Input: part model. Units: mm. Frame: model coordinates. A direction names the side the tool comes from. Round coordinates to 2 decimals unless told otherwise and drop trailing zeros. Loops run counter-clockwise (first coordinate to the right, second up) from the corner with the lowest first, then second, coordinate; pieces in that order, holes last. Notation, with made-up numbers: M 63.5,29.5 L 120.5,29.5 A18 cw 120.5,57.5 Z; hole C 38.25,26.5 d7. An arc over 180 degrees is marked long. Return JSON: item names as keys, results as strings. Group by question number.
1) Section A-A (y = 21.75). Output: boundary loops of the cut face in (x, z), plus the area to 3 significant figures.
2) Section C-C (x = -21). Output: boundary loops of the cut face in (y, z), plus the area to 3 significant figures.
3) Material intervals for line 1 (Y direction, x = -4.25, z = 12); line 2 (Z direction, x = -4.25, y = 11.25); line 3 (Z direction, x = -14.75, y = 13), sorted ascending. Write a range as from..to.
4) Mould query, pull axis Z, two halves, no side actions, for faces 1 (the face through (-8, 14, 0)), 2 (the face through (-15, 0, -7)), 3 (the face through (-12, 13, -15)). Classes: +Z half, -Z half, draft (parallel to the pull), parting line (faces both ways), or undercut.
5) Section B-B (y = 13.5). Output: boundary loops of the cut face in (x, z).
6) Section D-D (x = -14.75). Output: boundary loops of the cut face in (y, z).
7) Access query for faces 4 (the face through (-22.25, 3.45, -0.15)), 5 (the face through (-25, 13, 0)), 6 (the face through (-6.1, 24, -1.2)). Directions: +Z, -Z, +X, -X, +Y, -Y. A direction counts if a zero-diameter tool reaches every point of the face in a straight line with its end or side. Return the directions, or none.
from build123d import *

# Parameters (mm, degrees)
SKETCH1_R            = 7
SKETCH1_R_2          = 2.75
SKETCH1_R_3          = 3.659852489
BOSS_EXTRUDE1_DEPTH  = 7
SKETCH2_R            = 8
SKETCH2_R_2          = 6
BOSS_EXTRUDE2_DEPTH  = 17
FILLET1_R            = 3
FILLET2_R            = 3
SKETCH3_R            = 1
SKETCH5_W            = 50
SKETCH5_H            = 30
BOSS_EXTRUDE3_DEPTH  = 27
SKETCH6_R            = 2
CUT_EXTRUDE1_DEPTH   = 57
INTERSECT3_OUTLINE_W = 27
INTERSECT3_OUTLINE_H = 30
INTERSECT3_OUTLINE_R = 2
INTERSECT3_DEPTH     = 25


with BuildPart() as part:
    # Sketch1 → Boss-Extrude1 (new body)
    with BuildSketch(Plane(origin=(0, 0, 0), x_dir=(1, 0, 0), z_dir=(0, 1, 0))):
        with BuildLine():
            ThreePointArc((-15.634333704, 6.748663161), (-22.25, 0), (-15.634333704, -6.748663161))
            ThreePointArc((-15.634333704, -6.748663161), (-12.054001616, -7.488359295), (-8.978814065, -9.465516285))
            ThreePointArc((-8.978814065, -9.465516285), (-0.448762307, -12.99442036), (8.273320847, -9.971141939))
            ThreePointArc((8.273320847, -9.971141939), (11.493139678, -8.165901558), (15.148520579, -7.651784261))
            ThreePointArc((15.148520579, -7.651784261), (23.159852489, 0), (15.148520579, 7.651784261))
            ThreePointArc((15.148520579, 7.651784261), (11.493139678, 8.165901558), (8.273320847, 9.971141939))
            ThreePointArc((8.273320847, 9.971141939), (-0.448762307, 12.99442036), (-8.978814065, 9.465516285))
            ThreePointArc((-8.978814065, 9.465516285), (-12.054001616, 7.488359295), (-15.634333704, 6.748663161))
        make_face()
        with Locations(Location((0, 0, 0), (0, 0, 270))):
            Circle(SKETCH1_R, mode=Mode.SUBTRACT)
        with Locations(Location((-15.5, 0, 0), (0, 0, 270))):
            Circle(SKETCH1_R_2, mode=Mode.SUBTRACT)
        with Locations(Location((15.5, 0, 0), (0, 0, 270))):
            Circle(SKETCH1_R_3, mode=Mode.SUBTRACT)
    extrude(amount=BOSS_EXTRUDE1_DEPTH)

    # Sketch2 → Boss-Extrude2 (add)
    with BuildSketch(Plane(origin=(0, 7, 0), x_dir=(1, 0, 0), z_dir=(0, 1, 0))):
        with Locations(Location((0, 0, 0), (0, 0, 270))):
            Circle(SKETCH2_R)
        with Locations(Location((0, 0, 0), (0, 0, 270))):
            Circle(SKETCH2_R_2, mode=Mode.SUBTRACT)
    extrude(amount=BOSS_EXTRUDE2_DEPTH)

    # Fillet1
    # the kernel refuses this fillet: 3 mm, written as the material it adds along each edge
    with BuildSketch(Plane(origin=(0, 7, 0), x_dir=(0, 0, 1), z_dir=(-1, 0, 0))) as fillet1_piece_1:
        with BuildLine():
            CenterArc((4, -2.236067977), FILLET1_R, 0, 48.189685104)
            Line((6, 0), (6.04, 0.04472136))
            ThreePointArc((6.04, 0.04472136), (6.5, 0.06), (7, 0.06))
            Line((7, 0.06), (7.06, 0))
            Line((7.06, 0), (7.06, -2.236067977))
            Line((7.06, -2.236067977), (7, -2.236067977))
        make_face()
    revolve(axis=Axis((0, 7, 0), (0, 1, 0)))
    with BuildSketch(Plane(origin=(0, 7, 0), x_dir=(0, 0, 1), z_dir=(-1, 0, 0))) as fillet1_piece_2:
        with BuildLine():
            CenterArc((8 + FILLET1_R, FILLET1_R), FILLET1_R, 180, 90)
            Line((8, FILLET1_R), (8 - FILLET1_R * 0.02, FILLET1_R))
            Line((8 - FILLET1_R * 0.02, FILLET1_R), (8 - FILLET1_R * 0.02, -FILLET1_R * 0.02))
            Line((8 - FILLET1_R * 0.02, -FILLET1_R * 0.02), (8 + FILLET1_R, -FILLET1_R * 0.02))
            Line((8 + FILLET1_R, -FILLET1_R * 0.02), (8 + FILLET1_R, 0))
        make_face()
    revolve(axis=Axis((0, 7, 0), (0, 1, 0)))

    # Fillet2
    fillet2_edges = [part.edges().sort_by_distance(p)[0] for p in [
        (0, 7, -6),
    ]]
    fillet(fillet2_edges, radius=FILLET2_R)


with BuildPart() as body_2:
    # Sketch3 → Revolve1 (revolve)
    with BuildSketch(Plane(origin=(0, 0, 0), x_dir=(0, 0, -1), z_dir=(1, 0, 0))):
        with Locations((8.5, 19.608844607)):
            Circle(SKETCH3_R)
    revolve(axis=Axis((0, 0, 0), (0, 1, 0)))


with BuildPart() as part_1:
    add(part.part)

    # Intersect1: read off the stored shape, not the designer's step
    # Intersect1: cut body 2
    add(body_2.part, mode=Mode.SUBTRACT)


with BuildPart() as body_2_2:
    # Sketch5 → Boss-Extrude3 (new body)
    with BuildSketch(Plane(origin=(0, 0, 0), x_dir=(-1, 0, 0), z_dir=(0, -1, 0))):
        Rectangle(SKETCH5_W, SKETCH5_H)
    extrude(amount=-BOSS_EXTRUDE3_DEPTH)

    # Sketch6 → Cut-Extrude1 (cut)
    with BuildSketch(Plane.ZY.offset(25)):
        with Locations((-11.920412871, 13.5)):
            Circle(SKETCH6_R)
        with Locations(Location((11.920412871, 13.5, 0), (0, 0, 180))):
            Circle(SKETCH6_R)
    extrude(amount=-CUT_EXTRUDE1_DEPTH, mode=Mode.SUBTRACT)

    # Intersect2: read off the stored shape, not the designer's step
    # Intersect2: cut part
    add(part_1.part, mode=Mode.SUBTRACT)

    # Intersect3: read off the stored shape, not the designer's step
    # Intersect3 outline → Intersect3 (cut)
    with BuildSketch(Plane.YZ):
        with Locations((13.5, 0)):
            Rectangle(INTERSECT3_OUTLINE_W, INTERSECT3_OUTLINE_H)
        with Locations((13.5, -11.920412871)):
            Circle(INTERSECT3_OUTLINE_R, mode=Mode.SUBTRACT)
        with Locations((13.5, 11.920412871)):
            Circle(INTERSECT3_OUTLINE_R, mode=Mode.SUBTRACT)
    extrude(amount=INTERSECT3_DEPTH, mode=Mode.SUBTRACT)


solid = body_2_2.part
Returned:
{
 "1": {"outline": "M -25,-15 L 0,-15 L 0,-8 A8 cw 0,8 L 0,15 L -25,15 Z; M 0,-6 L 0,6 A6 ccw Z", "area": "706 mm^2"},
 "2": {"outline": "M 0,-15 L 27,-15 L 27,15 L 0,15 L 0,3.91 L 7,3.91 L 7,-3.91 L 0,-3.91 Z; hole C 13.5,-11.92 d4; hole C 13.5,11.92 d4", "area": "730 mm^2"},
 "3": {"line 1": "y = 7..11.5, 15.5..27", "line 2": "z = -15..-6.78, -4.24..4.24, 6.78..15", "line 3": "z = -15..-13.86, -9.98..9.98, 13.86..15"},
 "4": {"face 1": "undercut", "face 2": "draft", "face 3": "-Z half"},
 "5": {"outline": "M -25,-15 L 0,-15 L 0,-13.92 L -25,-13.92 Z; M -25,-9.92 L 0,-9.92 L 0,-8 A8 cw 0,8 L 0,9.92 L -25,9.92 Z; M -25,13.92 L 0,13.92 L 0,15 L -25,15 Z; M 0,-6 L 0,6 A6 ccw Z"},
 "6": {"outline": "M 0,-15 L 27,-15 L 27,15 L 0,15 L 0,6.81 L 7,6.81 L 7,2.65 L 0,2.65 L 0,-2.65 L 7,-2.65 L 7,-6.81 L 0,-6.81 Z; hole C 13.5,-11.92 d4; hole C 13.5,11.92 d4"},
 "7": {"face 4": "-Y", "face 5": "+Z, -Z, -X, +Y, -Y", "face 6": "none"}
}
